Verification items for this drawing (mm, ordinates from the low corner). Round coordinates to 2 decimals unless told otherwise and drop trailing zeros. Loops run counter-clockwise (first coordinate to the right, second up) from the corner with the lowest first, then second, coordinate; pieces in that order, holes last. Notation, with made-up numbers: M 42,-23 L 57,-23 A24 cw 57,3 Z; hole C 62.25,33.5 d6. An arc over 180 degrees is marked long. One line per item, written item: value.
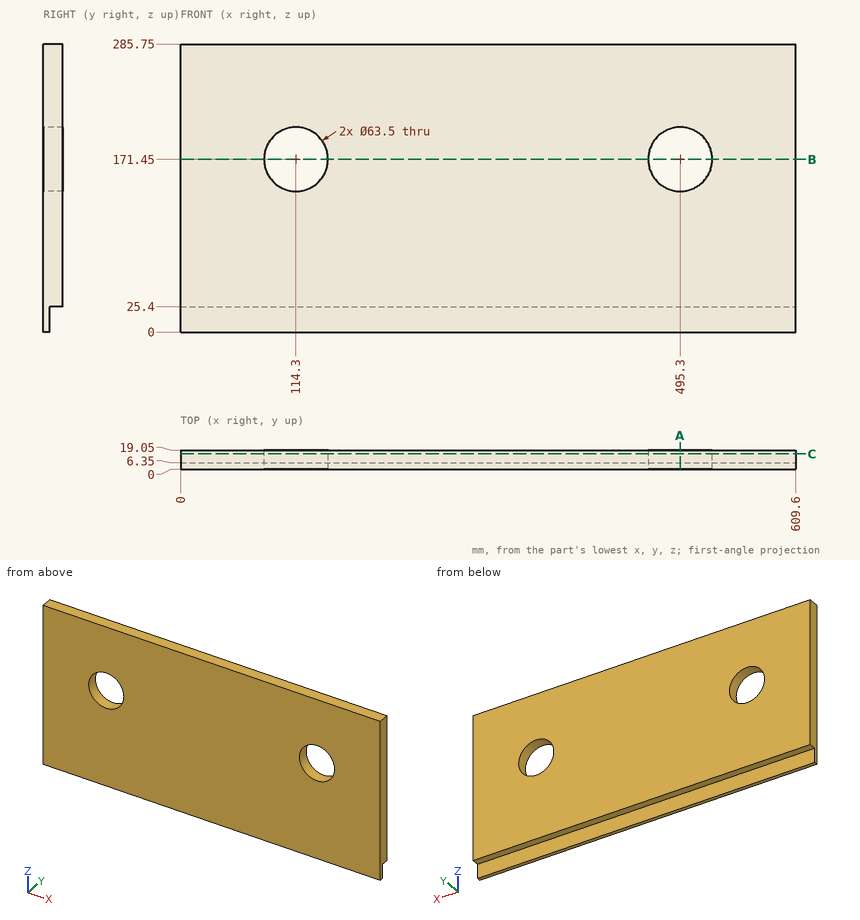
(1) Depth check by flat-ended pin: pin 1 Ø10 at (x, y) = (218.5, 14.5) entering from -Z; pin 2 Ø12.5 at (x, z) = (181, 17.5) entering from +Y. Enter the tip coordinate at first touch or a pass-through.
Completed:
pin 1: stops at z = 25.4
pin 2: stops at y = 6.35
(2) Sectioned sample at A-A on x = 495.3. Enter the section's corners in (y, z).
Completed:
outline: M 0,0 L 6.35,0 L 6.35,25.4 L 19.05,25.4 L 19.05,139.7 L 0,139.7 Z; M 0,203.2 L 19.05,203.2 L 19.05,285.75 L 0,285.75 Z
(3) Sectioned sample at B-B on z = 171.45. Enter the section's corners in (x, y).
Completed:
outline: M 0,0 L 82.55,0 L 82.55,19.05 L 0,19.05 Z; M 146.05,0 L 463.55,0 L 463.55,19.05 L 146.05,19.05 Z; M 527.05,0 L 609.6,0 L 609.6,19.05 L 527.05,19.05 Z
(4) Thickness scan on L1, parallel to X at y = 15, z = 172.5; L2, parallel to Z at x = 495.3, y = 13.5; L3, parallel to Z at x = 495.3, y = 5.75. Record the ranges inside material, lowest first. Write a range as from..to.
Completed:
L1: x = 0..82.57, 146.03..463.57, 527.03..609.6
L2: z = 25.4..139.7, 203.2..285.75
L3: z = 0..139.7, 203.2..285.75
(5) Sectioned sample at C-C on y = 15.5. Enter the section's corners in (x, z), and give its area (3 significant figures).
Completed:
outline: M 0,25.4 L 609.6,25.4 L 609.6,285.75 L 0,285.75 Z; hole C 114.3,171.45 d63.5; hole C 495.3,171.45 d63.5
area: 152,000 mm^2
